Read the model definition and answer for the solid it produces. Units are mm, in the model's axes. A direction names the side the tool comes from. Give positions to 0.01 mm unless a question says otherwise; leave off trailing zeros. Loops run counter-clockwise (first coordinate to the right, second up) from the corner with the lowest first, then second, coordinate; pieces in that order, holes last. Notation, with made-up numbers: (-37, 6.5) - (-10, 6.5) arc R11 ccw to (-10, 21.5) - close; hole circle Ø2 at (31, 81). An arc over 180 degrees is marked (long way). Put each result on its own line as item: value. Start each with the question number.
1. For a pull along X with two mould halves and no side action, classify faces 5 (the flat face through (-8.425, 0, 8)), 6 (the flat face through (0, 0, -3.175)), 7 (the flat face through (0, 3.25, 10)), 8 (the flat face through (-5.25, 0, 10)) as released by +X, released by -X, zero draft, split by the parting line, or undercut.
2. A cutting plane is placed at B-B, the plane y = 4. Determine the outline of the cut face in (x, z) (3 decimals), plus the area to 3 significant figures.
3. A cutting plane is placed at A-A, the plane z = 0.5. Determine the outline of the cut face in (x, y) (3 decimals).
4. Given pin 1 Ø5 at (x, y) = (-1, 0) entering from +Z; pin 2 Ø1.6 at (x, y) = (0, 5.5) entering from +Z, each flat-ended and moving along its own axis, determine where each tip first touches the part or whether it passes through.
5. A cutting plane is placed at D-D, the plane y = -0.5. Determine the outline of the cut face in (x, z) (3 decimals), plus the area to 3 significant figures.
6. Consider L1, parallel to X at y = 4.25, z = 6 (3 decimals); L2, parallel to Y at x = 1.5, z = 0.25 (3 decimals); L3, parallel to X at y = 5.75, z = 16.25 (3 decimals). Determine where each line is inside the solid, lowest interval first. Write a range as from..to.
7. A cutting plane is placed at C-C, the plane x = 0. Determine the outline of the cut face in (y, z) (3 decimals), plus the area to 3 significant figures.
8. For faces 1 (the flat face through (0, 5, 15.84)), 2 (the flat face through (0, -6.425, 8)), 3 (the cylindrical face through (-1.15, 4.86, 8.77)), 4 (the flat face through (0, -3.25, 10)), determine the directions among +Z, -Z, +X, -X, +Y, -Y from which every point of the face is accessible in a straight line to the end or side of a thin tool.
```python
from build123d import *

# Parameters (mm, degrees)
SKETCH1_W           = 10.5
SKETCH1_H           = 6.5
BOSS_EXTRUDE1_DEPTH = 19.84
SHELL1_T            = 3.175
CUT_EXTRUDE1_REACH  = 27.094
SKETCH2_R           = 3
SKETCH2_W           = 10.5
SKETCH2_H           = 4


with BuildPart() as part:
    # Sketch1 → Boss-Extrude1 (new body)
    with BuildSketch(Plane.XY):
        Rectangle(SKETCH1_W, SKETCH1_H)
    extrude(amount=BOSS_EXTRUDE1_DEPTH)

    # Shell1
    shell1_openings = [part.faces().sort_by_distance(p)[0] for p in [
        (0, 0, 19.84),
    ]]
    offset(amount=SHELL1_T, openings=shell1_openings, kind=Kind.INTERSECTION)

    # Sketch2 → Cut-Extrude1 (cut, up to next)
    with BuildSketch(Plane(origin=(0, 6.425, 0), x_dir=(1, 0, 0), z_dir=(0, 1, 0)), mode=Mode.PRIVATE) as cut_extrude1_sk1:
        with Locations(Location((0, -6, 0), (0, 0, 270))):
            Circle(SKETCH2_R)
    cut_extrude1_tool1 = extrude(cut_extrude1_sk1.sketch, amount=-CUT_EXTRUDE1_REACH, mode=Mode.PRIVATE) & part.part
    # Sketch2 → Cut-Extrude1 (cut, up to next)
    with BuildSketch(Plane(origin=(0, 6.425, 0), x_dir=(1, 0, 0), z_dir=(0, 1, 0)), mode=Mode.PRIVATE) as cut_extrude1_sk2:
        with Locations((0, -17.84)):
            Rectangle(SKETCH2_W, SKETCH2_H)
    cut_extrude1_tool2 = extrude(cut_extrude1_sk2.sketch, amount=-CUT_EXTRUDE1_REACH, mode=Mode.PRIVATE) & part.part
    add(cut_extrude1_tool1.solids().sort_by_distance((0, 6.425, 6))[0], mode=Mode.SUBTRACT)
    add(cut_extrude1_tool2.solids().sort_by_distance((0, 6.425, 17.84))[0], mode=Mode.SUBTRACT)


solid = part.part
```
Return value:
1. face 5: released by -X
1. face 6: zero draft
1. face 7: undercut
1. face 8: undercut
2. outline: (-8.425, -3.175) - (8.425, -3.175) - (8.425, 19.84) - (5.25, 19.84) - (5.25, 15.84) - (-5.25, 15.84) - (-5.25, 19.84) - (-8.425, 19.84) - close; hole circle Ø6 at (0, 6)
2. area: 318 mm2
3. outline: (-8.425, -6.425) - (8.425, -6.425) - (8.425, 6.425) - (-8.425, 6.425) - close; hole (-5.25, -3.25) - (5.25, -3.25) - (5.25, 3.25) - (-5.25, 3.25) - close
4. pin 1: stops at z = 0
4. pin 2: stops at z = 15.84
5. outline: (-8.425, -3.175) - (8.425, -3.175) - (8.425, 19.84) - (5.25, 19.84) - (5.25, 0) - (-5.25, 0) - (-5.25, 19.84) - (-8.425, 19.84) - close
5. area: 179 mm2
6. L1: x = -8.425..-3, 3..8.425
6. L2: y = -6.425..-3.25, 3.25..6.425
6. L3: x = -8.425..-5.25, 5.25..8.425
7. outline: (-6.425, -3.175) - (6.425, -3.175) - (6.425, 3) - (3.25, 3) - (3.25, 0) - (-3.25, 0) - (-3.25, 19.84) - (-6.425, 19.84) - close; (3.25, 9) - (6.425, 9) - (6.425, 15.84) - (3.25, 15.84) - close
7. area: 135 mm2
8. face 1: +Z, +Y
8. face 2: +Z, -Z, +X, -X, -Y
8. face 3: +Y
8. face 4: +Z
